Can you work these out from the model? Positions are in its coordinate system, mm. Round coordinates to 2 decimals unless told otherwise and drop trailing zeros. Loops run counter-clockwise (first coordinate to the right, second up) from the corner with the lowest first, then second, coordinate; pieces in that order, holes last. Notation, with made-up numbers: (3, 43) -> (60, 43) arc R23 cw to (60, 62) -> close; hole circle Ø4 at (-8.5, 32). An arc over 180 degrees is marked (long way). Write each question's results on one line, items separated by ' | '.
from build123d import *

# Parameters (mm, degrees)
BOSS_EXTRUDE1_DEPTH   = 1
CHAMFER1_SIZE         = 0.5
CHAMFER1_SIZE2        = 1.743707222
CHAMFER1_PART_2_SIZE  = 0.5
CHAMFER1_PART_2_SIZE2 = 1.743707222
FILLET1_R             = 0.5
SKETCH2_R             = 1
CUT_EXTRUDE1_DEPTH    = 1
FILLET2_R             = 0.5
SKETCH3_R             = 1.5
CUT_EXTRUDE2_DEPTH    = 0.5


with BuildPart() as part:
    # Sketch1 → Boss-Extrude1 (new body)
    with BuildSketch(Plane.XY):
        Polygon((-6, -1.5), (-6, 0), (6, 0), (6, -1.5), (4.25, -1.5), (4.25, -3.5), (6, -3.5), (6, -5), (13.5, -5), (13.5, 5), (-13.5, 5), (-13.5, -5), (-6, -5), (-6, -3.5), (-4.25, -3.5), (-4.25, -1.5), align=None)
    extrude(amount=BOSS_EXTRUDE1_DEPTH)

    # Chamfer1
    chamfer1_edges = [part.edges().sort_by_distance(p)[0] for p in [
        (4.25, -3.5, 0.5),
        (4.25, -1.5, 0.5),
    ]]
    chamfer1_side = [part.faces().sort_by_distance(p)[0] for p in [
        (4.25, -2.5, 0.5),
    ]]
    chamfer(chamfer1_edges, length=CHAMFER1_SIZE, length2=CHAMFER1_SIZE2, reference=chamfer1_side[0])

    # Chamfer1 part 2
    chamfer1_part_2_edges = [part.edges().sort_by_distance(p)[0] for p in [
        (-4.25, -1.5, 0.5),
        (-4.25, -3.5, 0.5),
    ]]
    chamfer1_part_2_side = [part.faces().sort_by_distance(p)[0] for p in [
        (-4.25, -2.5, 0.5),
    ]]
    chamfer(chamfer1_part_2_edges, length=CHAMFER1_PART_2_SIZE, length2=CHAMFER1_PART_2_SIZE2, reference=chamfer1_part_2_side[0])

    # Fillet1
    fillet1_edges = [part.edges().sort_by_distance(p)[0] for p in [
        (4.25, -2, 0.5),
        (4.25, -3, 0.5),
        (-4.25, -2, 0.5),
        (-4.25, -3, 0.5),
    ]]
    fillet(fillet1_edges, radius=FILLET1_R)

    # Sketch2 → Cut-Extrude1 (cut)
    with BuildSketch(Plane.XY.offset(1)):
        with Locations((-7, 3)):
            Circle(SKETCH2_R)
        with Locations((7, 3)):
            Circle(SKETCH2_R)
    extrude(amount=-CUT_EXTRUDE1_DEPTH, mode=Mode.SUBTRACT)

    # Fillet2
    fillet2_edges = [part.edges().sort_by_distance(p)[0] for p in [
        (6, -5, 0.5),
        (6, 0, 0.5),
        (-6, 0, 0.5),
        (-6, -5, 0.5),
        (-13.5, -5, 0.5),
        (-13.5, 5, 0.5),
        (13.5, 5, 0.5),
        (13.5, -5, 0.5),
    ]]
    fillet(fillet2_edges, radius=FILLET2_R)

    # Sketch3 → Cut-Extrude2 (cut)
    with BuildSketch(Plane.XY.offset(1)):
        with Locations((-7, 3)):
            Circle(SKETCH3_R)
        with Locations((7, 3)):
            Circle(SKETCH3_R)
    extrude(amount=-CUT_EXTRUDE2_DEPTH, mode=Mode.SUBTRACT)


solid = part.part
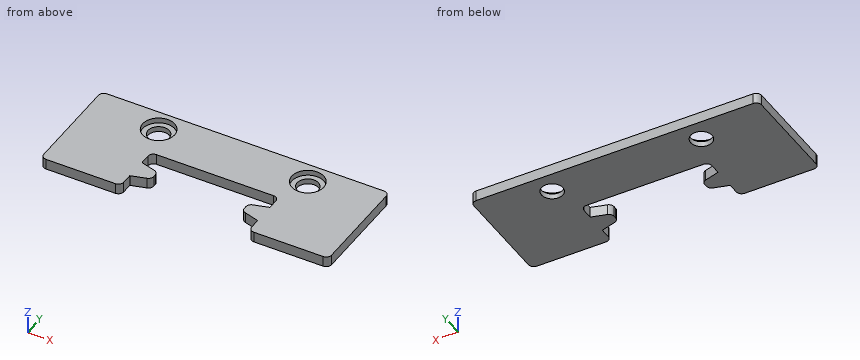
1. If we section it at B-B (z = 0.8): State how many separate pieces and enclosed holes the cut face has, then the cut area to 3 significant figures.
Final values:
separate pieces: 1 | enclosed holes: 2 | area: 201 mm2
2. If we section it at D-D (y = 3): List the corners of the cut face in (x, z) for me, then the cut area to 3 significant figures.
Final values:
outline: (-13.5, 0) -> (-8, 0) -> (-8, 0.5) -> (-8.5, 0.5) -> (-8.5, 1) -> (-13.5, 1) -> close; (-6, 0) -> (6, 0) -> (6, 0.5) -> (5.5, 0.5) -> (5.5, 1) -> (-5.5, 1) -> (-5.5, 0.5) -> (-6, 0.5) -> close; (8, 0) -> (13.5, 0) -> (13.5, 1) -> (8.5, 1) -> (8.5, 0.5) -> (8, 0.5) -> close | area: 22.0 mm2
3. Please list where these lines run through material, in increasing order: line 1 (X direction, y = 2.25, z = 0.3); line 2 (X direction, y = -3.75, z = 0.8); line 3 (Y direction, x = 7, z = 0.1). Write a range as from..to.
Final values:
line 1: -13.5..-7.66, -6.34..6.34, 7.66..13.5 | line 2: -13.5..-6, 6..13.5 | line 3: -5..2, 4..5
4. If we section it at A-A (y = -1): List the corners of the cut face in (x, z) for me.
Final values:
outline: (-13.5, 0) -> (-6, 0) -> (-6, 1) -> (-13.5, 1) -> close; (6, 0) -> (13.5, 0) -> (13.5, 1) -> (6, 1) -> close
5. If we section it at C-C (x = 7): List the corners of the cut face in (y, z) for me.
Final values:
outline: (-5, 0) -> (2, 0) -> (2, 0.5) -> (1.5, 0.5) -> (1.5, 1) -> (-5, 1) -> close; (4, 0) -> (5, 0) -> (5, 1) -> (4.5, 1) -> (4.5, 0.5) -> (4, 0.5) -> close
6. Will these pins go through, and if not, where does the flat tip stop? pin 1 (1.8 mm diameter, centred on x = 7, y = 3, fed in from +Z); pin 2 (2.5 mm diameter, centred on x = 7, y = 3, fed in from +Z); pin 3 (3.5 mm diameter, centred on x = -7, y = 3, fed in from +Z).
Final values:
pin 1: through | pin 2: z = 0.5 | pin 3: z = 1
